The model under review builds one solid part; all positions refer to its coordinate system, in mm. Face numbers are marked on the shaded views. Round coordinates to 2 decimals unless told otherwise and drop trailing zeros. Order: outer loops, then holes, each group sorted by start corner. A loop starts at its lowest first (then second) coordinate and runs counter-clockwise, first axis right, second up. Notation, with made-up numbers: (64, 5) -> (84, 5) arc R9 ccw to (84, 13) -> close; hole circle Ø6 at (81.25, 82.25). An arc over 180 degrees is marked (long way). Use a Markdown table: item, result. Add a question column.
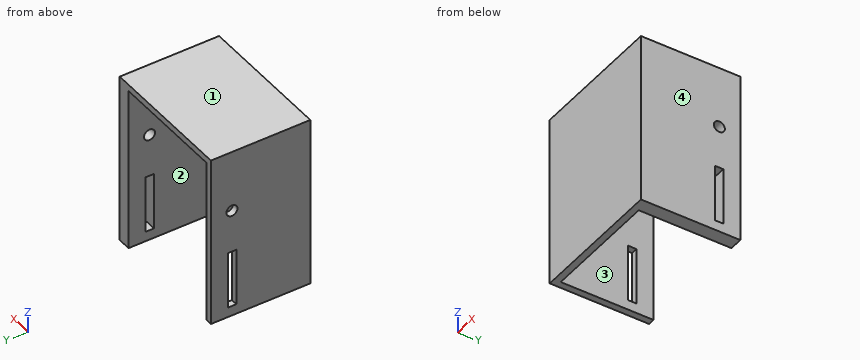
Autodesk Inventor part; units mm, degrees
ref_plane "YZ Plane" through (0, 0, 0) normal (1, 0, 0) x (0, 1, 0)
ref_plane "XZ Plane" through (0, 0, 0) normal (0, 1, 0) x (-1, 0, 0)
ref_plane "XY Plane" through (0, 0, 0) normal (0, 0, 1) x (1, 0, 0)
sketch "Sketch2" plane through (0, 0, 0) normal (0, 1, 0) x (-1, 0, 0)
  line L0 (0, 0) -> (-59, 0)
  line L1 (-59, 0) -> (-59, 78)
  line L2 (-59, 78) -> (0, 78)
  line L3 (0, 78) -> (0, 0)
  dimension "d0" = 59
  dimension "d1" = 78
extrude "Extrusion1" add sketch "Sketch2" along normal blind 45
shell "Shell1" thickness 3 removed faces 1 at (39.3333, 45, 52)
sketch "Sketch4" plane through (59, 0, 0) normal (0, 0, -1) x (-1, 0, 0)
  point P0 (59, 0)
sketch "Sketch5" plane through (3, 3, 3) normal (0, 0, 1) x (1, 0, 0)
  line L0 (0, 0) -> (0, 42)
  line L1 (0, 42) -> (53, 42)
  line L2 (0, 0) -> (53, 0)
  line L3 (53, 0) -> (53, 42)
  line L4 (53, 42) -> (0, 42)
  line L5 (0, 42) -> (0, 0)
  point P0 (-3, -3)
extrude "Extrusion3" cut sketch "Sketch5" against normal blind 10
sketch "Sketch6" plane through (0, 0, 0) normal (-1, 0, 0) x (0, 0, 1)
  line L0 (4.5, 37.3) -> (30.5, 37.3)
  line L1 (30.5, 37.3) -> (30.5, 33.5)
  line L2 (30.5, 33.5) -> (4.5, 33.5)
  line L3 (4.5, 33.5) -> (4.5, 37.3)
  line L4 (0, 0) -> (0, 45)
  line L5 (0, 0) -> (78, 0)
  dimension "d19" = 26
  dimension "d20" = 3.8
  dimension "d21" = 4.5
  dimension "d22" = 33.5
sketch "Sketch7" plane through (59, 0, 78) normal (1, 0, 0) x (0, 0, -1)
  line L0 (0, 0) -> (78, 0)
  line L1 (0, 45) -> (78, 45)
  line L2 (78, 45) -> (78, 0)
  line L3 (78, 0) -> (0, 0)
  line L4 (0, 0) -> (0, 45)
extrude "Extrusion5" add sketch "Sketch7" along normal blind 3
extrude "Extrusion6" cut sketch "Sketch6" against normal through all
sketch "Sketch8" plane through (0, 0, 0) normal (-1, 0, 0) x (0, 0, 1)
  circle A0 centre (50, 35.5) radius 2.5
  point P0 (0, 0)
  dimension "d29" = 5
extrude "Extrusion7" cut sketch "Sketch8" against normal through all
properties part number "arduino with shield box v06"
Q1. Draft analysis for pull direction X (two halves, no side actions). For the marked faces 1, 2, 3 and 4, state which applies: released by +X, released by -X, zero draft, split by the parting line, or undercut.
Q2. Add section A-A, the plane z = 50. Give the boundary of the cut face in (x, y), then the cut area to 3 significant figures.
Q3. To check wall thickness, follow line 1 along X through (y, z) = (5, 70); line 2 along Y through (x, z) = (1.15, 50); line 3 along Y through (x, z) = (56.5, 7). State the ranges of each line that lie inside material, in increasing order.
Q4. Add section B-B, the plane x = 58. Give the boundary of the cut face in (y, z).
Q5. For pin 1 (0.9 mm diameter, centred on x = 1.5, y = 35.5, fed in from -Z); pin 2 (21 mm diameter, centred on x = 30, y = 24.5, fed in from -Z); pin 3 (16 mm diameter, centred on x = 20, z = 32.5, fed in from +Y), all flat-tipped, find the tip position at first contact; note any pin that passes through.
Q6. Add section C-C, the plane y = 35.5. Give the boundary of the cut face in (x, z).
Q7. Add section D-D, the plane z = 11.5. Give the boundary of the cut face in (x, y), then the cut area to 3 significant figures.
Return value:
| question | item | result |
|---|---|---|
| 1 | face 1 | zero draft |
| 1 | face 2 | undercut |
| 1 | face 3 | undercut |
| 1 | face 4 | released by +X |
| 2 | outline | (0, 0) -> (62, 0) -> (62, 33) -> (56, 33) -> (56, 3) -> (3, 3) -> (3, 33) -> (0, 33) -> close; (0, 38) -> (3, 38) -> (3, 45) -> (0, 45) -> close; (56, 38) -> (62, 38) -> (62, 45) -> (56, 45) -> close |
| 2 | area | 519 mm² |
| 3 | line 1 | 0 to 3, 56 to 62 |
| 3 | line 2 | 0 to 33, 38 to 45 |
| 3 | line 3 | 0 to 33.5, 37.3 to 45 |
| 4 | outline | (0, 0) -> (45, 0) -> (45, 78) -> (0, 78) -> close; hole circle Ø5 at (35.5, 50); hole (33.5, 4.5) -> (37.3, 4.5) -> (37.3, 30.5) -> (33.5, 30.5) -> close |
| 5 | pin 1 | z = 0 |
| 5 | pin 2 | z = 75 |
| 5 | pin 3 | y = 3 |
| 6 | outline | (0, 0) -> (3, 0) -> (3, 4.5) -> (0, 4.5) -> close; (0, 30.5) -> (3, 30.5) -> (3, 47.5) -> (0, 47.5) -> close; (0, 52.5) -> (3, 52.5) -> (3, 75) -> (56, 75) -> (56, 52.5) -> (62, 52.5) -> (62, 78) -> (0, 78) -> close; (56, 0) -> (62, 0) -> (62, 4.5) -> (56, 4.5) -> close; (56, 30.5) -> (62, 30.5) -> (62, 47.5) -> (56, 47.5) -> close |
| 7 | outline | (0, 0) -> (62, 0) -> (62, 33.5) -> (56, 33.5) -> (56, 3) -> (3, 3) -> (3, 33.5) -> (0, 33.5) -> close; (0, 37.3) -> (3, 37.3) -> (3, 45) -> (0, 45) -> close; (56, 37.3) -> (62, 37.3) -> (62, 45) -> (56, 45) -> close |
| 7 | area | 530 mm² |
